```python
from build123d import *

# Parameters (mm, degrees)
SKETCH1_W           = 95
SKETCH1_H           = 23.5
BOSS_EXTRUDE1_DEPTH = 3
SKETCH2_R           = 6
CUT_EXTRUDE1_DEPTH  = 4
SKETCH4_W           = 3
SKETCH4_H           = 5
BOSS_EXTRUDE2_DEPTH = 3
SKETCH9_W           = 3
SKETCH9_H           = 39
BOSS_EXTRUDE5_DEPTH = 21.5
CUT_EXTRUDE5_DEPTH  = 4
FILLET5_R           = 5
LPATTERN1_COUNT     = 3
LPATTERN1_PITCH     = 35


with BuildPart() as part:
    # Sketch1 → Boss-Extrude1 (new body)
    with BuildSketch(Plane(origin=(0, 0, 0), x_dir=(0, 0, -1), z_dir=(1, 0, 0))):
        with Locations((17.5, 11.75)):
            Rectangle(SKETCH1_W, SKETCH1_H)
    extrude(amount=BOSS_EXTRUDE1_DEPTH)

    # Sketch2 → Cut-Extrude1 (cut, through all)
    with BuildSketch(Plane(origin=(3, 0, 0), x_dir=(0, 0, -1), z_dir=(1, 0, 0))):
        with Locations((6.8, 23.5)):
            Circle(SKETCH2_R)
    extrude(amount=-CUT_EXTRUDE1_DEPTH, mode=Mode.SUBTRACT)

    # Sketch4 → Boss-Extrude2 (add)
    with BuildSketch(Plane.XZ):
        with Locations((1.5, 17.5)):
            Rectangle(SKETCH4_W, SKETCH4_H)
    boss_extrude2 = extrude(amount=BOSS_EXTRUDE2_DEPTH)

    # Sketch9 → Boss-Extrude5 (add)
    with BuildSketch(Plane(origin=(0, 23.5, 0), x_dir=(1, 0, 0), z_dir=(0, 1, 0))):
        with Locations((1.5, 45.5)):
            Rectangle(SKETCH9_W, SKETCH9_H)
    extrude(amount=BOSS_EXTRUDE5_DEPTH)

    # Sketch10 → Cut-Extrude5 (cut, through all)
    with BuildSketch(Plane(origin=(3, 0, 0), x_dir=(0, 0, -1), z_dir=(1, 0, 0))):
        with BuildLine():
            Line((39.3, 35), (39.3, 45))
            Line((39.3, 45), (49.3, 45))
            Line((49.3, 45), (49.3, 35))
            ThreePointArc((49.3, 35), (44.3, 30), (39.3, 35))
        make_face()
    extrude(amount=-CUT_EXTRUDE5_DEPTH, mode=Mode.SUBTRACT)

    # Fillet5
    fillet5_edges = [part.edges().sort_by_distance(p)[0] for p in [
        (1.5, 45, -26),
        (1.5, 45, -65),
        (1.5, 23.5, 30),
    ]]
    fillet(fillet5_edges, radius=FILLET5_R)

    # LPattern1: Boss-Extrude2 ×3
    with Locations(*[(0, 0, -i * LPATTERN1_PITCH) for i in range(1, LPATTERN1_COUNT)]):
        add(boss_extrude2)


solid = part.part
```
For this review, take the finished solid that the model builds, in its own axes (mm). A direction names the side the tool comes from. Coordinates: 2 decimals unless noted, no trailing zeros. Order: outer loops, then holes, each group sorted by start corner. A loop starts at its lowest first (then second) coordinate and runs counter-clockwise, first axis right, second up. Notation, with made-up numbers: (68, 9) - (75, 9) arc R20 ccw to (75, 14) - close; hole circle Ø7 at (-2.75, -29). An arc over 180 degrees is marked (long way). Answer as a JSON object with one key per item and string values. Group by question number.
1. The part is to be moulded in two halves that separate along Z. For faces 1 (the flat face through (1, 0, 0)), 2 (the cylindrical face through (2, 43, -64)), 3 (the cylindrical face through (1.52, 22.07, 28.5)), 4 (the flat face through (1, 45, -35)), say which applies: pulls with the +Z half, pulls with the -Z half, needs draft (parallel to the pull), parting line crosses it, or undercut.
2. Clearance check with flat-ended pins moving along their axes: P1, Ø1.5, axis at x = 2, y = 38, coming from the +Z side; P2, Ø1.5, axis at x = 1, z = 26, coming from the -Y side; P3, Ø0.9, axis at x = 2, z = -18, coming from the +Y side. State where each tip first meets the part, or that it passes through.
3. We need section B-B on z = 13. State the section outline as (x, y) points.
4. For probe 1 along Z at (x, y) = (1.7, 36.5); probe 2 along Y at (x, z) = (0.55, 13); probe 3 along Z at (x, y) = (0.7, 20), list the stretches that pass through material, from the lowest coordinate up.
5. For faces 5 (the flat face through (2, 40, -39.3)), 6 (the flat face through (1, 23.5, -19)), 7 (the flat face through (1, -1, -55)), list the 3-axis set-ups (+Z, -Z, +X, -X, +Y, -Y) from which the entire face can be reached by the end or side of a thin tool; tool diameter is ignored.
6. We need section C-C on y = 27.5. State the section outline as (x, z) points, then the cut area to 3 significant figures.
7. We need section A-A on x = 2.5. State the section outline as (y, z) points.
Final values:
{
 "1": {"face 1": "undercut", "face 2": "pulls with the -Z half", "face 3": "pulls with the +Z half", "face 4": "needs draft"},
 "2": {"P1": "z = -26", "P2": "y = 0", "P3": "y = 23.5"},
 "3": {"outline": "(0, 0) - (3, 0) - (3, 23.5) - (0, 23.5) - close"},
 "4": {"probe 1": "-65 to -49.3, -39.3 to -26", "probe 2": "0 to 23.5", "probe 3": "-65 to -11.67, -1.93 to 29.77"},
 "5": {"face 5": "+X, -X, +Y", "face 6": "+Z, +X, -X, +Y", "face 7": "-Z, +X, -X, -Y"},
 "6": {"outline": "(0, -65) - (3, -65) - (3, -26) - (0, -26) - close", "area": "117 mm²"},
 "7": {"outline": "(-3, -55) - (0, -55) - (0, -65) - (40, -65) arc R5 ccw to (45, -60) - (45, -49.3) - (35, -49.3) arc R5 cw to (35, -39.3) - (45, -39.3) - (45, -31) arc R5 ccw to (40, -26) - (23.5, -26) - (23.5, -12.8) arc R6 cw to (23.5, -0.8) - (23.5, 25) arc R5 ccw to (18.5, 30) - (0, 30) - (0, 20) - (-3, 20) - (-3, 15) - (0, 15) - (0, -15) - (-3, -15) - (-3, -20) - (0, -20) - (0, -50) - (-3, -50) - close"}
}
